Geometry: final body of the model. Coordinates: model frame, mm. A direction names the side the tool comes from. Coordinates: 2 decimals unless noted, no trailing zeros. Loops run counter-clockwise (first coordinate to the right, second up) from the corner with the lowest first, then second, coordinate; pieces in that order, holes last. Notation, with made-up numbers: (77, 44.25) - (110, 44.25) arc R24 cw to (110, 74.25) - close; hole circle Ø4 at (-35, 25). An arc over 180 degrees is marked (long way). Write each question's results on one line, items separated by ' | '. Start each with the question number.
Solid Edge part; units mm, degrees
sketch "Sketch1" plane through (0, 0, 0) normal (0, -1, 0) x (1, 0, 0)
  arc A0 (-37.1299, 86.2147) -> (92.6101, -40.7853) centre (-39.0034, -45.4688) cw
  line L0 (92.6101, -40.7853) -> (92.6101, -101.2453)
  line L1 (92.6101, -101.2453) -> (95.6101, -101.2453)
  line L2 (95.6101, -101.2453) -> (95.6101, -40.7853)
  arc A1 (-37.1299, 89.2147) -> (95.6101, -40.7853) centre (-39.0019, -45.4657) cw
  line L3 (-97.1299, 89.2147) -> (-37.1299, 89.2147)
  line L4 (-97.1299, 86.2147) -> (-97.1299, 89.2147)
  line L5 (-37.1299, 86.2147) -> (-97.1299, 86.2147)
  dimension "D1" = 37.1299
  dimension "D2" = 92.6101
  dimension "D3" = 37.1299
  dimension "D4" = 95.6101
extrude "Protrusion1" add sketch "Sketch1" against normal blind 170
sketch "Sketch2" plane through (-67.1299, 85, 89.2147) normal (0, 0, 1) x (1, 0, 0)
  circle A0 centre (-5, 57.5) radius 3
  circle A1 centre (-5, -57.5) radius 3
extrude "Cutout1" cut sketch "Sketch2" against normal through all
sketch "Sketch3" plane through (95.6101, 85, -66.0153) normal (1, 0, 0) x (0, 1, 0)
  circle A0 centre (58, -10.23) radius 3
  circle A1 centre (-58, -10.23) radius 3
  dimension "D1" = 58
extrude "Cutout2" cut sketch "Sketch3" against normal through all
properties material "Nylon, allgemein"
1) Pull-direction query (Y, two-part tool) for faces 1 (the flat face through (64, 170, 37)), 2 (the flat face through (-67, 84, 86.215)), 3 (the flat face through (64, 0, 37)), 4 (the cylindrical face through (-70.52, 145.03, 87.74)); classes: released by +Y, released by -Y, zero draft, split by the parting line, or undercut.
2) Section query A-A on y = 124. Output: boundary loops of the cut face in (x, z).
3) Material intervals for line 1 (X direction, y = 28, z = -60); line 2 (Z direction, x = -66, y = 58); line 3 (Z direction, x = 17, y = 32), sorted ascending. Write a range as [from, to].
4) Section query C-C on x = -80. Output: boundary loops of the cut face in (y, z), and give its area (3 significant figures).
5) Pin query (flat end, axial travel): pin 1 Ø12 at (x, y) = (2, 61.5) entering from +Z; pin 2 Ø12 at (x, y) = (61.5, 31.5) entering from +Z; pin 3 Ø12 at (x, y) = (-28, 47) entering from +Z. Return the tip coordinate at first contact, or that it passes through.
6) Section query B-B on z = -69. Output: boundary loops of the cut face in (x, y).
7) Access query for faces 5 (the flat face through (92.61, 84, -71)), 6 (the cylindrical face through (56.26, 83.81, 49.76)). Directions: +Z, -Z, +X, -X, +Y, -Y. A direction counts if a zero-diameter tool reaches every point of the face in a straight line with its end or side. Return the directions, or none.
Returned:
1) face 1: released by +Y | face 2: zero draft | face 3: released by -Y | face 4: undercut
2) outline: (-97.13, 86.21) - (-37.13, 86.21) arc R131.7 cw to (92.61, -40.79) - (92.61, -101.25) - (95.61, -101.25) - (95.61, -40.79) arc R134.69 ccw to (-37.13, 89.21) - (-97.13, 89.21) - close
3) line 1: x = [92.61, 95.61] | line 2: z = [86.21, 89.21] | line 3: z = [73.73, 77.03]
4) outline: (0, 86.21) - (170, 86.21) - (170, 89.21) - (0, 89.21) - close | area: 510 mm²
5) pin 1: stops at z = 84.6 | pin 2: stops at z = 50.51 | pin 3: stops at z = 89.13
6) outline: (92.61, 0) - (95.61, 0) - (95.61, 170) - (92.61, 170) - close
7) face 5: -Z, -X, +Y, -Y | face 6: +Z, +X, +Y, -Y
